from build123d import *

# Parameters (mm, degrees)
SKETCH1_W           = 40
SKETCH1_H           = 40
BOSS_EXTRUDE1_DEPTH = 10.66
SKETCH2_R           = 19
CUT_EXTRUDE1_DEPTH  = 1
CUT_EXTRUDE2_START  = -1
SKETCH3_R           = 19
CUT_EXTRUDE2_DEPTH  = 1
SKETCH4_R           = 1.785
CUT_EXTRUDE3_DEPTH  = 58.564186783
CUT_EXTRUDE4_DEPTH  = 3.25
CHAMFER1_SIZE       = 0.5
FILLET1_R           = 4


with BuildPart() as part:
    # Sketch1 → Boss-Extrude1 (new body)
    with BuildSketch(Plane(origin=(0, 0, 0), x_dir=(1, 0, 0), z_dir=(0, 1, 0))):
        with Locations((-20, 20)):
            Rectangle(SKETCH1_W, SKETCH1_H)
    extrude(amount=BOSS_EXTRUDE1_DEPTH)

    # Sketch2 → Cut-Extrude1 (cut)
    with BuildSketch(Plane(origin=(0, 10.66, 0), x_dir=(1, 0, 0), z_dir=(0, 1, 0))):
        with Locations(Location((-20, 20, 0), (0, 0, 270))):
            Circle(SKETCH2_R)
    extrude(amount=-CUT_EXTRUDE1_DEPTH, mode=Mode.SUBTRACT)

    # Sketch3 → Cut-Extrude2 (cut)
    with BuildSketch(Plane.XZ.offset(CUT_EXTRUDE2_START)):
        with Locations(Location((-20, -20, 0), (0, 0, 90))):
            Circle(SKETCH3_R)
    extrude(amount=CUT_EXTRUDE2_DEPTH, mode=Mode.SUBTRACT)

    # Sketch4 → Cut-Extrude3 (cut, through all)
    with BuildSketch(Plane(origin=(0, 10.66, 0), x_dir=(1, 0, 0), z_dir=(0, 1, 0))):
        with Locations(Location((-36.25, 36.25, 0), (0, 0, 270))):
            Circle(SKETCH4_R)
        with Locations(Location((-3.75, 36.25, 0), (0, 0, 270))):
            Circle(SKETCH4_R)
        with Locations(Location((-3.75, 3.75, 0), (0, 0, 270))):
            Circle(SKETCH4_R)
        with Locations(Location((-36.25, 3.75, 0), (0, 0, 270))):
            Circle(SKETCH4_R)
    extrude(amount=-CUT_EXTRUDE3_DEPTH, mode=Mode.SUBTRACT)

    # Sketch5 → Cut-Extrude4 (cut)
    with BuildSketch(Plane.XZ):
        Polygon((-39.019012185, -34.626083484), (-39.040859049, -37.836076638), (-36.271846864, -39.459993154), (-33.480987815, -37.873916516), (-33.459140951, -34.663923362), (-36.228153136, -33.040006846), align=None)
        Polygon((-34.626083484, -0.980987815), (-37.836076638, -0.959140951), (-39.459993154, -3.728153136), (-37.873916516, -6.519012185), (-34.663923362, -6.540859049), (-33.040006846, -3.771846864), align=None)
        Polygon((-5.373916516, -39.019012185), (-2.163923362, -39.040859049), (-0.540006846, -36.271846864), (-2.126083484, -33.480987815), (-5.336076638, -33.459140951), (-6.959993154, -36.228153136), align=None)
        Polygon((-0.980987815, -5.373916516), (-0.959140951, -2.163923362), (-3.728153136, -0.540006846), (-6.519012185, -2.126083484), (-6.540859049, -5.336076638), (-3.771846864, -6.959993154), align=None)
    extrude(amount=-CUT_EXTRUDE4_DEPTH, mode=Mode.SUBTRACT)

    # Chamfer1
    chamfer1_edges = [part.edges().sort_by_distance(p)[0] for p in [
        (-36.25, 10.66, -5.535),
        (-3.75, 10.66, -5.535),
        (-3.75, 10.66, -38.035),
        (-36.25, 10.66, -38.035),
    ]]
    chamfer(chamfer1_edges, length=CHAMFER1_SIZE)

    # Fillet1
    fillet1_edges = [part.edges().sort_by_distance(p)[0] for p in [
        (0, 5.33, 0),
        (-40, 5.33, 0),
        (-40, 5.33, -40),
        (0, 5.33, -40),
    ]]
    fillet(fillet1_edges, radius=FILLET1_R)


solid = part.part
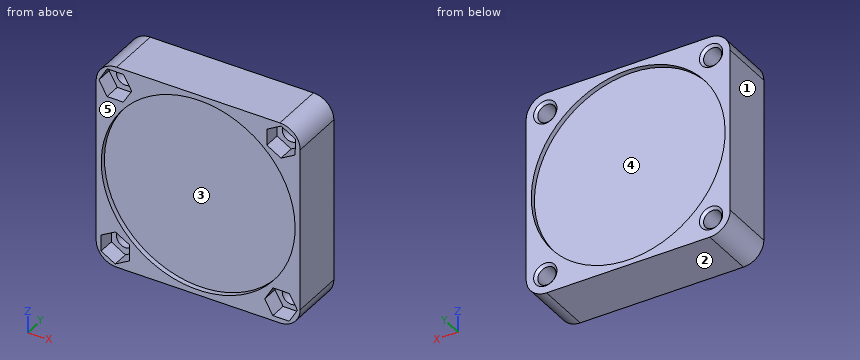
The listing builds one solid part. Answer for the finished solid, in the listing's coordinates (mm). Face numbers are marked on the shaded views. A direction names the side the tool comes from. Coordinates: 2 decimals unless noted, no trailing zeros. Write each loop counter-clockwise with the first axis right and the second up, starting at its lowest first coordinate (ties: lowest second). Pieces come first, ordered by that corner, then holes. Notation, with made-up numbers: (-19.5, 22.25) - (-3.5, 22.25) arc R12 ccw to (-3.5, 28.25) - close; hole circle Ø1 at (73.5, 86). An arc over 180 degrees is marked (long way). Answer as CSV lines item,"result".
1. Find section A-A (y = 0.5). Give the number of separate pieces and of enclosed holes in the cut face, plus the area to 3 significant figures.
Computed values:
separate pieces,"1"
enclosed holes,"5"
area,"345 mm²"
2. Find section B-B (x = -20). Give the vertices of the cut face in (y, z).
Computed values:
outline,"(0, -40) - (10.66, -40) - (10.66, -39) - (9.66, -39) - (9.66, -1) - (10.66, -1) - (10.66, 0) - (0, 0) - (0, -1) - (1, -1) - (1, -39) - (0, -39) - close"
3. Given P1, Ø1.7, axis at x = -37.5, z = -36.5, coming from the -Y side; P2, Ø3, axis at x = -38, z = -5, coming from the -Y side; P3, Ø4, axis at x = -6.5, z = -13, coming from the +Y side; P4, Ø5, axis at x = -13, z = -17, coming from the -Y side, each flat-ended and moving along its own axis, determine where each tip first touches the part or whether it passes through.
Computed values:
P1,"stops at y = 3.25"
P2,"stops at y = 0"
P3,"stops at y = 9.66"
P4,"stops at y = 1"
4. A tool of negligible diameter and unlimited length cuts with its end or side. For the marked faces 4 and 5, from which of +Z, -Z, +X, -X, +Y, -Y can it reach the whole face along a straight path? Write none if from no direction.
Computed values:
face 4,"+Y"
face 5,"+Z, -Z, +X, -X, -Y"
5. Straight lines are drawn through the part: line 1 (X direction, y = 8.75, z = -36.5); line 2 (X direction, y = 0.8, z = -20); line 3 (Y direction, x = -11, z = -34). For each, find the intervals that lie inside material, in ascending order. Write a range as [from, to].
Computed values:
line 1,"x = [-39.97, -38.02], [-34.48, -5.52], [-1.98, -0.03]"
line 2,"x = [-40, -39], [-1, 0]"
line 3,"y = [1, 9.66]"
6. Find section C-C (z = -20). Give the vertices of the cut face in (x, y).
Computed values:
outline,"(-40, 0) - (-39, 0) - (-39, 1) - (-1, 1) - (-1, 0) - (0, 0) - (0, 10.66) - (-1, 10.66) - (-1, 9.66) - (-39, 9.66) - (-39, 10.66) - (-40, 10.66) - close"
7. Determine the mould class of the marked faces 1, 2 and 3 for opening direction X: +X half, -X half, draft (parallel to the pull), parting line (faces both ways), or undercut.
Computed values:
face 1,"-X half"
face 2,"draft"
face 3,"undercut"
8. Find section D-D (y = 5). Give the vertices of the cut face in (x, z) (3 decimals).
Computed values:
outline,"(-40, -36) arc R4 ccw to (-36, -40) - (-4, -40) arc R4 ccw to (0, -36) - (0, -4) arc R4 ccw to (-4, 0) - (-36, 0) arc R4 ccw to (-40, -4) - close; hole circle Ø3.57 at (-36.25, -36.25); hole circle Ø3.57 at (-36.25, -3.75); hole circle Ø3.57 at (-3.75, -36.25); hole circle Ø3.57 at (-3.75, -3.75)"
